Source: CAD feature listing. Evaluate the final solid. Frame: model axes, mm. Face numbers are marked on the shaded views. A direction names the side the tool comes from. Give positions to 0.01 mm unless a question says otherwise; leave off trailing zeros. Write each loop counter-clockwise with the first axis right and the second up, starting at its lowest first coordinate (ties: lowest second). Pieces come first, ordered by that corner, then holes. Notation, with made-up numbers: (0.5, 31) -> (12.5, 31) arc R28 ccw to (12.5, 61) -> close; hole circle Ø4 at (42.25, 60). An arc over 180 degrees is marked (long way). Answer as a JSON object with one key per item and string values. Group by question number.
Item 1: Access query for the marked faces 1 and 2. Directions: +Z, -Z, +X, -X, +Y, -Y. A direction counts if a zero-diameter tool reaches every point of the face in a straight line with its end or side. Return the directions, or none.
Item 2: Ray query, probe 1 along Y at (x, z) = (0, 4.5); probe 2 along Y at (x, z) = (0, 7). Return the intervals inside material, ascending. Write a range as from..to.
Item 3: Section query A-A on x = 0. Return the cut outline in (y, z).
Item 4: Section query D-D on z = 7.25. Return the cut outline in (x, y), plus the area to 3 significant figures.
Item 5: First-contact query: pin 1 Ø2 at (x, z) = (6, 8) entering from -Y; pin 2 Ø4 at (y, z) = (-2.5, 1.5) entering from -X; pin 3 Ø6 at (x, z) = (3.5, 2) entering from -Y. Flat tips, straight axial feed; report the tip coordinate or a pass-through.
Item 6: Section query B-B on y = -0.75. Return the cut outline in (x, z).
Item 7: Section query C-C on z = 2.25. Return the cut outline in (x, y), plus the area to 3 significant figures.
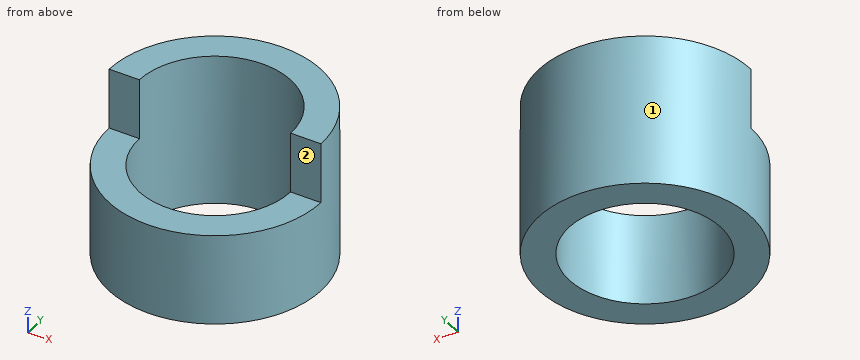
from build123d import *

# Parameters (mm, degrees)
SKETCH1_R           = 7
SKETCH1_R_2         = 5
BOSS_EXTRUDE1_DEPTH = 10
SKETCH3_W           = 4
SKETCH3_H           = 7
CUT_EXTRUDE1_DEPTH  = 10


with BuildPart() as part:
    # Sketch1 → Boss-Extrude1 (new body)
    with BuildSketch(Plane.XY):
        Circle(SKETCH1_R)
        Circle(SKETCH1_R_2, mode=Mode.SUBTRACT)
    extrude(amount=BOSS_EXTRUDE1_DEPTH)

    # Sketch3 → Cut-Extrude1 (cut, symmetric)
    with BuildSketch(Plane(origin=(0, 0, 0), x_dir=(0, 0, -1), z_dir=(1, 0, 0))):
        with Locations((-8, -3.5)):
            Rectangle(SKETCH3_W, SKETCH3_H)
    extrude(amount=CUT_EXTRUDE1_DEPTH, both=True, mode=Mode.SUBTRACT)


solid = part.part
Worked answers:
{
 "1": {"face 1": "+Z, -Z", "face 2": "+Z, +X, -X, -Y"},
 "2": {"probe 1": "-7..-5, 5..7", "probe 2": "5..7"},
 "3": {"outline": "(-7, 0) -> (-5, 0) -> (-5, 6) -> (-7, 6) -> close; (5, 0) -> (7, 0) -> (7, 10) -> (5, 10) -> close"},
 "4": {"outline": "(-7, 0) -> (-5, 0) arc R5 cw to (5, 0) -> (7, 0) arc R7 ccw to start", "area": "37.7 mm^2"},
 "5": {"pin 1": "y = 0", "pin 2": "x = -6.98", "pin 3": "y = -6.98"},
 "6": {"outline": "(-6.96, 0) -> (-4.94, 0) -> (-4.94, 6) -> (-6.96, 6) -> close; (4.94, 0) -> (6.96, 0) -> (6.96, 6) -> (4.94, 6) -> close"},
 "7": {"outline": "circle Ø14 at (0, 0); hole circle Ø10 at (0, 0)", "area": "75.4 mm^2"}
}
